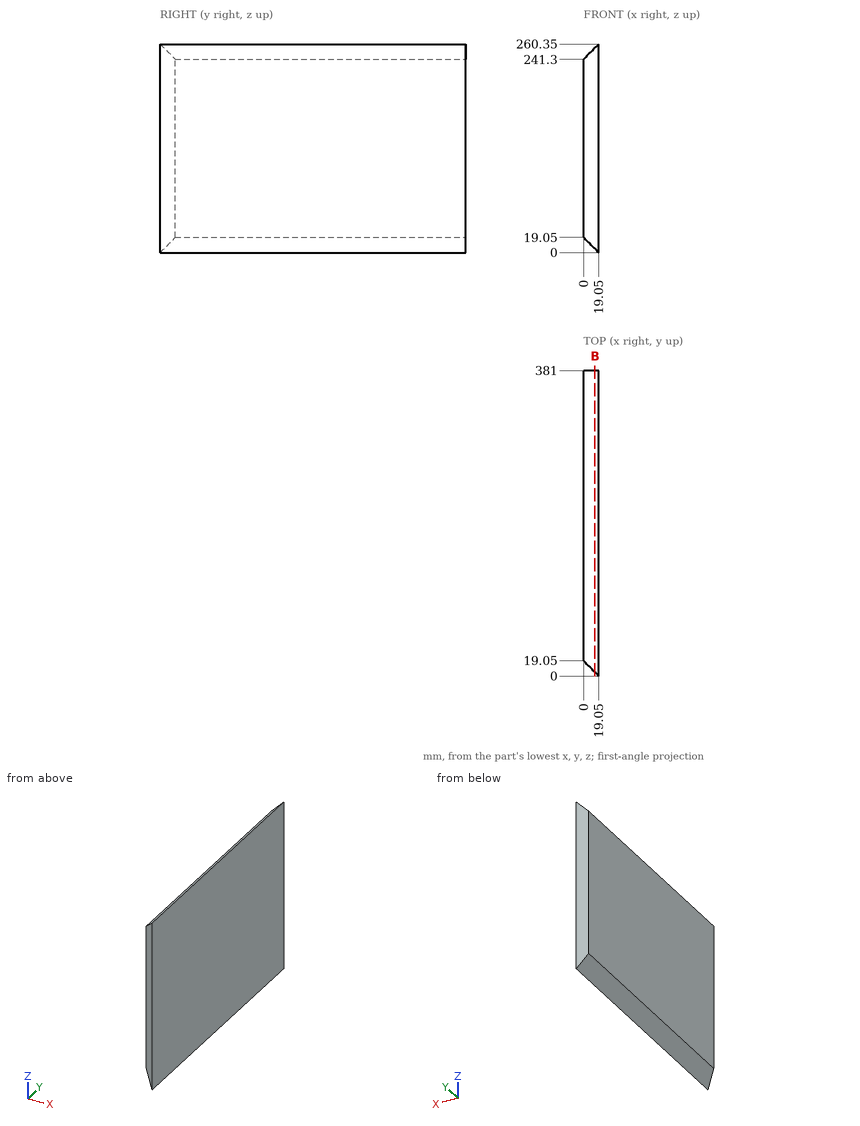
The figure shows three views and two pictorial views of one solid part (mm, origin at its lowest corner). Answer the questions. Coordinates: 2 decimals unless noted, no trailing zeros. Order: outer loops, then holes, each group sorted by start corner. A loop starts at its lowest first (then second) coordinate and runs counter-clockwise, first axis right, second up. Notation, with made-up numbers: (48.25, -3) - (95.25, -3) arc R20 cw to (95.25, 36) - close; hole circle Ø9 at (44, 89). An arc over 180 degrees is marked (long way). Answer as a JSON object with one key per item and string values.
1. Each of these flat-tipped pins is pushed along its axis until it touches: P1, Ø5, axis at x = 14, y = 296, coming from the +Z side; P2, Ø4, axis at x = 15.5, z = 220.5, coming from the -Y side; P3, Ø3, axis at x = 13, y = 160, coming from the -Z side. Where does it stop, or does it pass through?
Output values:
{"P1": "stops at z = 257.8", "P2": "stops at y = 1.55", "P3": "stops at z = 4.55"}
2. Find section B-B on x = 14.25. Determine the outline of the cut face in (y, z), plus the area to 3 significant figures.
Output values:
{"outline": "(4.8, 4.8) - (381, 4.8) - (381, 255.55) - (4.8, 255.55) - close", "area": "94,300 mm²"}
3. Consider line 1 (Y direction, x = 2.5, z = 201.5); line 2 (Z direction, x = 13, y = 164); line 3 (Z direction, x = 14.5, y = 157). Determine where each line is inside the solid, lowest interval first.
Output values:
{"line 1": "y = 16.55 to 381", "line 2": "z = 6.05 to 254.3", "line 3": "z = 4.55 to 255.8"}
